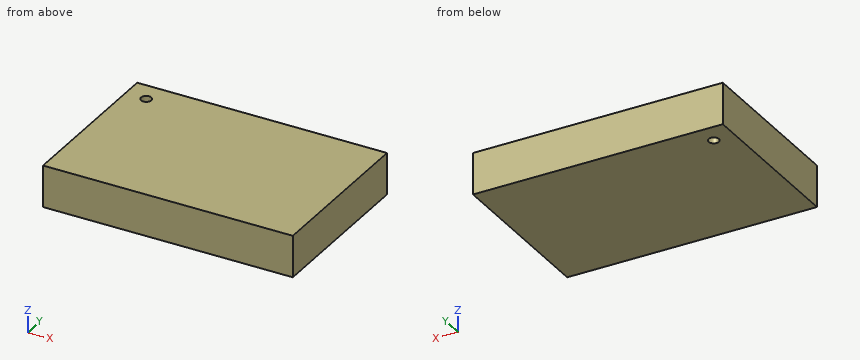
Autodesk Inventor part; units mm, degrees
ref_plane "YZ Plane" through (0, 0, 0) normal (1, 0, 0) x (0, 1, 0)
ref_plane "XZ Plane" through (0, 0, 0) normal (0, 1, 0) x (-1, 0, 0)
ref_plane "XY Plane" through (0, 0, 0) normal (0, 0, 1) x (1, 0, 0)
sketch "Sketch1" plane through (0, 0, 0) normal (0, 0, 1) x (1, 0, 0)
  line L0 (0, 0) -> (152.4, 0)
  line L1 (152.4, 0) -> (152.4, 101.6)
  line L2 (152.4, 101.6) -> (0, 101.6)
  line L3 (0, 101.6) -> (0, 0)
  dimension "d0" = 152.4
  dimension "d1" = 101.6
extrude "Extrusion1" add sketch "Sketch1" along normal blind 25.4
sketch "Sketch2" plane through (0, 0, 25.4) normal (0, 0, 1) x (1, 0, 0)
  line L0 (152.4, 101.6) -> (0, 101.6)
  line L1 (0, 101.6) -> (0, 0)
  circle A0 centre (12.7, 88.9) radius 3.175
  dimension "d4" = 6.35
  dimension "d5" = 12.7
  dimension "d6" = 12.7
extrude "Extrusion2" cut sketch "Sketch2" against normal through all
properties part number "Rectangular pattern"
Could you check a few things on this model? Use its own coordinates, in mm. Give positions to 0.01 mm unless a question says otherwise; leave off trailing zeros. Loops run counter-clockwise (first coordinate to the right, second up) from the corner with the lowest first, then second, coordinate; pieces in that order, holes last. Notation, with made-up numbers: (88, 42.25) - (110, 42.25) arc R17 cw to (110, 52.25) - close; hole circle Ø5 at (25.25, 56.5). An arc over 180 degrees is marked (long way). Use one line per item in the form item = value.
1. I'm going to push flat-ended pins straight in: pin 1 Ø1 at (y, z) = (26.5, 19.5) entering from -X; pin 2 Ø4 at (x, y) = (12.7, 88.9) entering from +Z. Where does each tip first touch, or does it pass through?
Response values:
pin_1 = 0
pin_2 = through
2. I need wall thicknesses on probe 1 along Y at (x, z) = (12.7, 7.25) (3 decimals); probe 2 along X at (y, z) = (90, 3.5). Which ranges of each line are inside material? Lowest first, please.
Response values:
probe_1 = 0 to 85.725, 92.075 to 101.6
probe_2 = 0 to 9.72, 15.68 to 152.4
3. I want a section at B-B (y = 88.9). Please give me the cut outline in (x, z) (3 decimals), and give its area (3 significant figures).
Response values:
outline = (0, 0) - (9.525, 0) - (9.525, 25.4) - (0, 25.4) - close; (15.875, 0) - (152.4, 0) - (152.4, 25.4) - (15.875, 25.4) - close
area = 3,710 mm²
4. I want a section at A-A (x = 12.7). Please give me the cut outline in (y, z) (3 decimals), and give its area (3 significant figures).
Response values:
outline = (0, 0) - (85.725, 0) - (85.725, 25.4) - (0, 25.4) - close; (92.075, 0) - (101.6, 0) - (101.6, 25.4) - (92.075, 25.4) - close
area = 2,420 mm²
